```python
from build123d import *

# Parameters (mm, degrees)
SKETCH1_W           = 80
SKETCH1_H           = 35
BOSS_EXTRUDE1_DEPTH = 2
BOSS_EXTRUDE2_DEPTH = 20
CUT_EXTRUDE1_DEPTH  = 2.3


with BuildPart() as part:
    # Sketch1 → Boss-Extrude1 (new body)
    with BuildSketch(Plane(origin=(0, 0, 0), x_dir=(1, 0, 0), z_dir=(0, 1, 0))):
        with Locations((40, -17.5)):
            Rectangle(SKETCH1_W, SKETCH1_H)
    extrude(amount=BOSS_EXTRUDE1_DEPTH)

    # Sketch2 → Boss-Extrude2 (add)
    with BuildSketch(Plane(origin=(0, 2, 0), x_dir=(1, 0, 0), z_dir=(0, 1, 0))):
        Polygon((0, 0), (80, 0), (80, -7.5), (76, -7.5), (76, -2), (4, -2), (4, -7.5), (0, -7.5), align=None)
        Polygon((0, -35), (80, -35), (80, -27.5), (76, -27.5), (76, -33), (4, -33), (4, -27.5), (0, -27.5), align=None)
    extrude(amount=BOSS_EXTRUDE2_DEPTH)

    # Sketch3 → Cut-Extrude1 (cut)
    with BuildSketch(Plane(origin=(0, 22, 0), x_dir=(1, 0, 0), z_dir=(0, 1, 0))):
        Polygon((2.490559859, -0.891238969), (1.285064709, -1.020782184), (0.794504851, -2.129543216), (1.509440141, -3.108761031), (2.714935291, -2.979217816), (3.205495149, -1.870456784), align=None)
        Polygon((2, -31.787564435), (0.95, -32.393782217), (0.95, -33.606217783), (2, -34.212435565), (3.05, -33.606217783), (3.05, -32.393782217), align=None)
        Polygon((78.304035901, -31.826304055), (77.135567446, -32.149849214), (76.831531545, -33.323545158), (77.695964099, -34.173695945), (78.864432554, -33.850150786), (79.168468455, -32.676454842), align=None)
        Polygon((78.932445098, -1.225050879), (77.795096923, -0.805004297), (76.862651826, -1.579953418), (77.067554902, -2.774949121), (78.204903077, -3.194995703), (79.137348174, -2.420046582), align=None)
    extrude(amount=-CUT_EXTRUDE1_DEPTH, mode=Mode.SUBTRACT)


solid = part.part
```
Geometry: final body of the model. Coordinates: model frame, mm. A direction names the side the tool comes from. Round coordinates to 2 decimals unless told otherwise and drop trailing zeros. Order: outer loops, then holes, each group sorted by start corner. A loop starts at its lowest first (then second) coordinate and runs counter-clockwise, first axis right, second up. Notation, with made-up numbers: (85, 70) -> (124, 70) arc R22 ccw to (124, 97) -> close; hole circle Ø7 at (87, 40.25). An arc over 180 degrees is marked (long way). Use CSV: the item, a comma, the result in double quotes. Start each with the question number.
1) Section D-D (z = 22). Return the cut outline in (x, y).
2) Section C-C (z = 6). Return the cut outline in (x, y).
3) Section A-A (y = 5.25). Return the cut outline in (x, z).
4) Material intervals for line 1 along Z through (x, y) = (9, 2.5); line 2 along X through (y, z) = (5.25, 7); line 3 along Y through (x, z) = (22, 19), sorted ascending. Write a range as from..to.
5) Section B-B (x = 72). Return the cut outline in (y, z), and give its area (3 significant figures).
6) First-contact query: pin 1 Ø1.9 at (x, z) = (78, 33) entering from +Y; pin 2 Ø9.5 at (x, z) = (21.5, 25) entering from +Y. Flat tips, straight axial feed; report the tip coordinate or a pass-through.
7) Set-up query: faces 4 (the face through (2, 19.7, 2)), 5 (the face through (78, 12, 27.5)), 6 (the face through (39.8, 22, 33.2)). Return all of +Z, -Z, +X, -X, +Y, -Y with unobstructed straight access to the full face (end or side cutting, diameter ignored); none if empty.
8) Draft query along X for faces 1 (the face through (0, 1, 18)), 2 (the face through (76, 12, 30)), 3 (the face through (2, 12, 27.5)). Return one class per face: +X half, -X half, draft (parallel to the pull), parting line (faces both ways), or undercut.
Returned:
1,outline,"(0, 0) -> (80, 0) -> (80, 2) -> (0, 2) -> close"
2,outline,"(0, 0) -> (80, 0) -> (80, 22) -> (76, 22) -> (76, 2) -> (4, 2) -> (4, 22) -> (0, 22) -> close"
3,outline,"(0, 0) -> (80, 0) -> (80, 7.5) -> (76, 7.5) -> (76, 2) -> (4, 2) -> (4, 7.5) -> (0, 7.5) -> close; (0, 27.5) -> (4, 27.5) -> (4, 33) -> (76, 33) -> (76, 27.5) -> (80, 27.5) -> (80, 35) -> (0, 35) -> close"
4,line 1,"z = 0..2, 33..35"
4,line 2,"x = 0..4, 76..80"
4,line 3,"y = 0..2"
5,outline,"(0, 0) -> (22, 0) -> (22, 2) -> (2, 2) -> (2, 33) -> (22, 33) -> (22, 35) -> (0, 35) -> close"
5,area,"150 mm²"
6,pin 1,"stops at y = 19.7"
6,pin 2,"stops at y = 2"
7,face 4,"+Y"
7,face 5,"+X, -X, +Y"
7,face 6,"+Z, -Z, +X, -X, +Y"
8,face 1,"-X half"
8,face 2,"undercut"
8,face 3,"draft"
